Here's how the part is built. I have some questions about the finished solid (model axes, mm). Coordinates: 2 decimals unless noted, no trailing zeros. Write each loop counter-clockwise with the first axis right and the second up, starting at its lowest first coordinate (ties: lowest second). Pieces come first, ordered by that corner, then holes. Notation, with made-up numbers: M -33.5,-3 L -15.5,-3 A21 ccw -15.5,36 Z; hole C -33,5 d1. An arc over 180 degrees is marked long. Use one line per item in the form item = value. Start each with the question number.
1. I want a section at A-A, the plane y = 13. List the corners of the cut face in (x, z) for me, plus the area to 3 significant figures.
2. I want a section at B-B, the plane z = 2.2. List the corners of the cut face in (x, y) for me.
3. I'm going to push flat-ended pins straight in: pin 1 Ø6 at (x, y) = (193, 2.5) entering from -Z; pin 2 Ø1.5 at (x, z) = (129.5, 1.5) entering from +Y. Where does each tip first touch, or does it pass through?
from build123d import *

# Parameters (mm, degrees)
SKETCH2_W           = 220
SKETCH2_H           = 20
BOSS_EXTRUDE1_DEPTH = 3
SKETCH4_W           = 3
SKETCH4_H           = 10
CUT_EXTRUDE2_DEPTH  = 221.927589947
LPATTERN1_COUNT     = 6
LPATTERN1_PITCH     = 40


with BuildPart() as part:
    # Sketch2 → Boss-Extrude1 (new body)
    with BuildSketch(Plane.XY):
        with Locations((110, 10)):
            Rectangle(SKETCH2_W, SKETCH2_H)
    extrude(amount=BOSS_EXTRUDE1_DEPTH)

    # Sketch4 → Cut-Extrude2 (cut, through all)
    with BuildSketch(Plane.XY):
        with Locations((10, 15)):
            Rectangle(SKETCH4_W, SKETCH4_H)
    cut_extrude2 = extrude(amount=CUT_EXTRUDE2_DEPTH, mode=Mode.SUBTRACT)

    # LPattern1: Cut-Extrude2 ×6
    with Locations(*[(i * LPATTERN1_PITCH, 0, 0) for i in range(1, LPATTERN1_COUNT)]):
        add(cut_extrude2, mode=Mode.SUBTRACT)


solid = part.part
Answer list:
q1.outline = M 0,0 L 8.5,0 L 8.5,3 L 0,3 Z; M 11.5,0 L 48.5,0 L 48.5,3 L 11.5,3 Z; M 51.5,0 L 88.5,0 L 88.5,3 L 51.5,3 Z; M 91.5,0 L 128.5,0 L 128.5,3 L 91.5,3 Z; M 131.5,0 L 168.5,0 L 168.5,3 L 131.5,3 Z; M 171.5,0 L 208.5,0 L 208.5,3 L 171.5,3 Z; M 211.5,0 L 220,0 L 220,3 L 211.5,3 Z
q1.area = 606 mm²
q2.outline = M 0,0 L 220,0 L 220,20 L 211.5,20 L 211.5,10 L 208.5,10 L 208.5,20 L 171.5,20 L 171.5,10 L 168.5,10 L 168.5,20 L 131.5,20 L 131.5,10 L 128.5,10 L 128.5,20 L 91.5,20 L 91.5,10 L 88.5,10 L 88.5,20 L 51.5,20 L 51.5,10 L 48.5,10 L 48.5,20 L 11.5,20 L 11.5,10 L 8.5,10 L 8.5,20 L 0,20 Z
q3.pin_1 = 0
q3.pin_2 = 10
